from build123d import *

# Parameters (mm, degrees)
BOSS_EXTRUDE3_DEPTH      = 3
BOSS_EXTRUDE3_DEPTH_BACK = 3
FILLET1_R                = 0.75
SKETCH5_W                = 55
SKETCH5_H                = 10
BOSS_EXTRUDE4_DEPTH      = 1
SKETCH6_R                = 1.65
CUT_EXTRUDE2_DEPTH       = 10
SKETCH7_R                = 1.5
CUT_EXTRUDE3_DEPTH       = 1
CUT_EXTRUDE4_REACH       = 32.087


with BuildPart() as part:
    # Sketch1 → Boss-Extrude3 (new, two sides: drawn at the far end of the back side and taken through both)
    with BuildSketch(Plane(origin=(0, 0, 0), x_dir=(1, 0, 0), z_dir=(0, 1, 0)).offset(-BOSS_EXTRUDE3_DEPTH_BACK)):
        with BuildLine():
            Line((27.5, 10), (-27.5, 10))
            Line((-27.5, 10), (-27.5, 6.45))
            Line((-27.5, 6.45), (-20.252630365, 6.45))
            ThreePointArc((-20.252630365, 6.45), (-14.2, 5), (-20.252630365, 3.55))
            Line((-20.252630365, 3.55), (-27.5, 3.55))
            Line((-27.5, 3.55), (-27.5, 0))
            Line((-27.5, 0), (27.5, 0))
            Line((27.5, 0), (27.5, 3.55))
            Line((27.5, 3.55), (20.252630365, 3.55))
            ThreePointArc((20.252630365, 3.55), (14.2, 5), (20.252630365, 6.45))
            Line((20.252630365, 6.45), (27.5, 6.45))
            Line((27.5, 6.45), (27.5, 10))
        make_face()
    extrude(amount=BOSS_EXTRUDE3_DEPTH + BOSS_EXTRUDE3_DEPTH_BACK)

    # Fillet1
    fillet1_edges = [part.edges().sort_by_distance(p)[0] for p in [
        (-20.252630365, 0, -6.45),
        (20.252630365, 0, -6.45),
        (20.252630365, 0, -3.55),
        (-20.252630365, 0, -3.55),
    ]]
    fillet(fillet1_edges, radius=FILLET1_R)

    # Sketch5 → Boss-Extrude4 (add)
    with BuildSketch(Plane(origin=(0, 3, 0), x_dir=(1, 0, 0), z_dir=(0, 1, 0))):
        with Locations((0, 5)):
            Rectangle(SKETCH5_W, SKETCH5_H)
    extrude(amount=BOSS_EXTRUDE4_DEPTH)

    # Sketch6 → Cut-Extrude2 (cut)
    with BuildSketch(Plane(origin=(0, 0, -10), x_dir=(-1, 0, 0), z_dir=(0, 0, -1))):
        with Locations((-10, 1)):
            Circle(SKETCH6_R)
        with Locations(Location((10, 1, 0), (0, 0, 180))):
            Circle(SKETCH6_R)
    extrude(amount=-CUT_EXTRUDE2_DEPTH, mode=Mode.SUBTRACT)

    # Sketch7 → Cut-Extrude3 (cut)
    with BuildSketch(Plane.XZ.offset(-3)):
        with Locations(Location((-17.4, -5, 0), (0, 0, 270))):
            Circle(SKETCH7_R)
        with Locations(Location((17.4, -5, 0), (0, 0, 270))):
            Circle(SKETCH7_R)
    extrude(amount=-CUT_EXTRUDE3_DEPTH, mode=Mode.SUBTRACT)

    # Cut-Extrude4: up to this face of the body (flat: up to its plane)
    cut_extrude4_end = Plane(part.part.faces().sort_by_distance((0, 4, -5))[0])
    # Sketch8 → Cut-Extrude4 (cut, up to the picked face)
    with BuildSketch(Plane.XZ.offset(3), mode=Mode.PRIVATE) as cut_extrude4_sk1:
        Polygon((-13.464101615, 0), (-10, -6), (10, -6), (13.464101615, 0), align=None)
    cut_extrude4_tool1 = split(extrude(cut_extrude4_sk1.sketch, amount=-CUT_EXTRUDE4_REACH, mode=Mode.PRIVATE), bisect_by=cut_extrude4_end, keep=Keep.BOTH, mode=Mode.PRIVATE)
    add(cut_extrude4_tool1.solids().sort_by(Axis((0, -3, -2.852366), (0, 1, 0)))[0], mode=Mode.SUBTRACT)


solid = part.part
CAD build for the part. Positions are in the model's coordinates, mm. A direction names the side the tool comes from. Give positions to 0.01 mm unless a question says otherwise; leave off trailing zeros. Loops run counter-clockwise (first coordinate to the right, second up) from the corner with the lowest first, then second, coordinate; pieces in that order, holes last. Notation, with made-up numbers: M 89,-34.5 L 138,-34.5 A10 ccw 138,-28.5 Z; hole C 56,34 d7. An arc over 180 degrees is marked long. Write each question's results on one line, items separated by ' | '.
Q1. Flat gauge pins, fed straight in: P1, Ø3, axis at x = -17, y = 3, coming from the +Z side; P2, Ø2, axis at x = 10, y = 1, coming from the +Z side; P3, Ø1.5, axis at x = -18, z = -6.5, coming from the -Y side; P4, Ø2, axis at x = 2, y = 1, coming from the +Z side. Where does each tip first touch, or does it go through?
Geometry check:
P1: stops at z = 0 | P2: passes through | P3: stops at y = 3 | P4: stops at z = -6
Q2. Which spindle directions (+Z, -Z, +X, -X, +Y, -Y) get a long thin tool onto all of the face, cutting with end or side? Do faces 1 (the face through (-12.14, 0.45, -2.29)), 2 (the face through (-24, 0, -6.45)), 3 (the face through (-14.2, 0, -5.1)), 4 (the face through (24, 0, -6.45)), 5 (the face through (20, 0, 0)). Say none if no direction does.
Geometry check:
face 1: +Z, +Y, -Y | face 2: -X, -Y | face 3: -Y | face 4: +X, -Y | face 5: +Z, +X, -X, +Y, -Y
Q3. Band-saw the part on D-D on z = -1.25. Write the cut outline in (x, y), and give its area (3 significant figures).
Geometry check:
outline: M -27.5,-3 L -12.74,-3 L -12.74,4 L -27.5,4 Z; M 12.74,-3 L 27.5,-3 L 27.5,4 L 12.74,4 Z | area: 207 mm²
Q4. Probe probe 1 along X at (y, z) = (-1, -2.5); probe 2 along X at (y, z) = (1, -5); probe 3 along X at (y, z) = (3.5, -5). List the from-to ranges inside material, lowest first.
Geometry check:
probe 1: x = -27.5 to -19.4, -15.4 to -12.02, 12.02 to 15.4, 19.4 to 27.5 | probe 2: x = -14.2 to -11.65, 11.65 to 14.2 | probe 3: x = -27.5 to -18.9, -15.9 to -10.58, 10.58 to 15.9, 18.9 to 27.5
Q5. Band-saw the part on C-C on x = 17.4. Write the cut outline in (y, z), and give its area (3 significant figures).
Geometry check:
outline: M -3,-10 L 4,-10 L 4,-6.5 L 3,-6.5 L 3,-8.2 L -3,-8.2 Z; M -3,-1.8 L 3,-1.8 L 3,-3.5 L 4,-3.5 L 4,0 L -3,0 Z | area: 28.6 mm²
Q6. Band-saw the part on B-B on z = -4.5. Write the cut outline in (x, y), and give its area (3 significant figures).
Geometry check:
outline: M -27.5,3 L -18.81,3 L -18.81,4 L -27.5,4 Z; M -15.99,3 L -14.24,3 L -14.24,-3 L -10.87,-3 L -10.87,-0.4 A1.65 cw -10.87,2.4 L -10.87,4 L -15.99,4 Z; M 10.87,-3 L 14.24,-3 L 14.24,3 L 15.99,3 L 15.99,4 L 10.87,4 L 10.87,2.4 A1.65 cw 10.87,-0.4 Z; M 18.81,3 L 27.5,3 L 27.5,4 L 18.81,4 Z | area: 65.0 mm²
Q7. Band-saw the part on A-A on y = 1. Write the cut outline in (x, z), and give its area (3 significant figures).
Geometry check:
outline: M -27.5,-10 L -11.65,-10 L -11.65,-3.14 L -13.46,0 L -27.5,0 L -27.5,-3.55 L -20.68,-3.55 A0.75 ccw -20.06,-3.22 A3.2 cw long -20.06,-6.78 A0.75 ccw -20.68,-6.45 L -27.5,-6.45 Z; M -8.35,-10 L 8.35,-10 L 8.35,-6 L -8.35,-6 Z; M 11.65,-10 L 27.5,-10 L 27.5,-6.45 L 20.68,-6.45 A0.75 ccw 20.06,-6.78 A3.2 cw long 20.06,-3.22 A0.75 ccw 20.68,-3.55 L 27.5,-3.55 L 27.5,0 L 13.46,0 L 11.65,-3.14 Z | area: 273 mm²
Q8. Mould opens along X. For faces 6 (the face through (-21, 3, -5)), 7 (the face through (-24, 0, -3.55)), 8 (the face through (-27.5, 0, -3)) say: pulls with the +X half, pulls with the -X half, needs draft (parallel to the pull), parting line crosses it, or undercut.
Geometry check:
face 6: undercut | face 7: needs draft | face 8: pulls with the -X half
